Source: CAD feature listing. Evaluate the final solid. Frame: model axes, mm. Face numbers are marked on the shaded views. A direction names the side the tool comes from. Give positions to 0.01 mm unless a question says otherwise; leave off trailing zeros. Order: outer loops, then holes, each group sorted by start corner. A loop starts at its lowest first (then second) coordinate and runs counter-clockwise, first axis right, second up.
1) Section A-A, the plane x = -37. Return loops of the section in (y, z).
2) Material intervals for line 1 (Y direction, x = -12, z = 0.9); line 2 (Y direction, x = 58, z = 1.5); line 3 (X direction, y = -35, z = 1.9), sorted ascending.
3) First-contact query: P1, Ø0.5, axis at y = 70.5, z = 1.5, coming from the -X side; P2, Ø0.8, axis at x = 70, z = 1.5, coming from the +Y side; P3, Ø0.5, axis at x = 73.5, z = 1.5, coming from the +Y side. Flat tips, straight axial feed; report the tip coordinate or a pass-through.
4) Access query for the marked faces 1 and 2. Directions: +Z, -Z, +X, -X, +Y, -Y. A direction counts if a zero-diameter tool reaches every point of the face in a straight line with its end or side. Return the directions, or none.
5) Section B-B, the plane z = 0.6. Return loops of the section in (x, y), plus the area to 4 significant figures.
6) Section C-C, the plane y = 20. Return loops of the section in (x, z), plus the area to 3 significant figures.
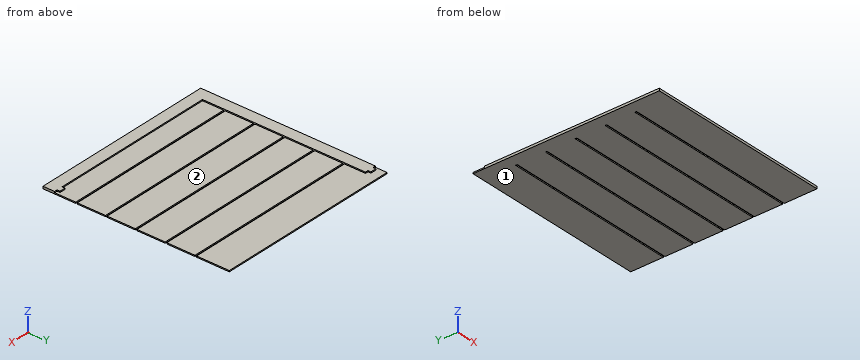
```python
from build123d import *

# Parameters (mm, degrees)
EXTRUDE_1_DEPTH = 1
EXTRUDE_2_DEPTH = 1


with BuildPart() as part:
    # 草图1 → 凸台-拉伸1 (new body)
    with BuildSketch(Plane.XY):
        Polygon((-75, 50.468617295), (-75, 51.868617295), (-65, 51.868617295), (75, 51.868617295), (75, 79.968617295), (-85, 79.968617295), (-85, -80.031382705), (75, -80.031382705), (75, -51.931382705), (-65, -51.931382705), (-75, -51.931382705), (-75, -50.531382705), (-65, -50.531382705), (75, -50.531382705), (75, -26.331382705), (-65, -26.331382705), (-75, -26.331382705), (-75, -24.931382705), (-65, -24.931382705), (75, -24.931382705), (75, -0.731382705), (-65, -0.731382705), (-75, -0.731382705), (-75, 0.668617295), (-65, 0.668617295), (75, 0.668617295), (75, 24.868617295), (-65, 24.868617295), (-75, 24.868617295), (-75, 26.268617295), (-65, 26.268617295), (75, 26.268617295), (75, 50.468617295), (-65, 50.468617295), align=None)
    extrude(amount=EXTRUDE_1_DEPTH)

    # 草图2 → 凸台-拉伸2 (add)
    with BuildSketch(Plane.XY.offset(1)):
        Polygon((-85, -80.031382705), (-85, -70.031382705), (-85, 69.968617295), (-82.5, 69.968617295), (-82.5, 72.468617295), (-77.5, 72.468617295), (-77.5, 69.968617295), (-75, 69.968617295), (-75, -70.031382705), (67.5, -70.031382705), (67.5, -67.531382705), (72.5, -67.531382705), (72.5, -70.031382705), (75, -70.031382705), (75, -80.031382705), align=None)
    extrude(amount=EXTRUDE_2_DEPTH)


solid = part.part
```
From the geometry:
1. outline: (-80.03, 0) - (-51.93, 0) - (-51.93, 1) - (-70.03, 1) - (-70.03, 2) - (-80.03, 2) - close; (-50.53, 0) - (-26.33, 0) - (-26.33, 1) - (-50.53, 1) - close; (-24.93, 0) - (-0.73, 0) - (-0.73, 1) - (-24.93, 1) - close; (0.67, 0) - (24.87, 0) - (24.87, 1) - (0.67, 1) - close; (26.27, 0) - (50.47, 0) - (50.47, 1) - (26.27, 1) - close; (51.87, 0) - (79.97, 0) - (79.97, 1) - (51.87, 1) - close
2. line 1: y = -80.03 to -51.93, -50.53 to -26.33, -24.93 to -0.73, 0.67 to 24.87, 26.27 to 50.47, 51.87 to 79.97
2. line 2: y = -80.03 to -70.03
2. line 3: x = -85 to -75
3. P1: stops at x = -82.5
3. P2: stops at y = -67.53
3. P3: stops at y = -70.03
4. face 1: -Z, +X, -X, +Y, -Y
4. face 2: +Z, +X, +Y
5. outline: (-85, -80.03) - (75, -80.03) - (75, -51.93) - (-75, -51.93) - (-75, -50.53) - (75, -50.53) - (75, -26.33) - (-75, -26.33) - (-75, -24.93) - (75, -24.93) - (75, -0.73) - (-75, -0.73) - (-75, 0.67) - (75, 0.67) - (75, 24.87) - (-75, 24.87) - (-75, 26.27) - (75, 26.27) - (75, 50.47) - (-75, 50.47) - (-75, 51.87) - (75, 51.87) - (75, 79.97) - (-85, 79.97) - close
5. area: 24,550 mm2
6. outline: (-85, 0) - (75, 0) - (75, 1) - (-75, 1) - (-75, 2) - (-85, 2) - close
6. area: 170 mm2
